from build123d import *

# Parameters (mm, degrees)
SKETCH_2_R      = 2
EXTRUDE_1_DEPTH = 5


with BuildPart() as part:
    # 草图2 → 凸台-拉伸1 (new, symmetric)
    with BuildSketch(Plane.XY):
        with BuildLine():
            ThreePointArc((18.5, 0), (15.999089719, 4.330652442), (10.99817977, 4.329075598))
            Line((10.99817977, 4.329075598), (2.50182023, 19.030924402))
            ThreePointArc((2.50182023, 19.030924402), (-1.295110422, 28.189356996), (0, 18.36))
            Line((0, 18.36), (0, 0))
            Line((0, 0), (-51.636977369, 0))
            Line((-51.636977369, 0), (-51.636977369, -8.430841873))
            Line((-51.636977369, -8.430841873), (41.612216194, -8.430841873))
            Line((41.612216194, -8.430841873), (41.612216194, 0))
            Line((41.612216194, 0), (18.5, 0))
        make_face()
        with BuildLine():
            ThreePointArc((15.280750547, 0), (13.5, -1.780750547), (11.719249453, 0))
            ThreePointArc((11.719249453, 0), (13.5, 1.780750547), (15.280750547, 0))
        make_face(mode=Mode.SUBTRACT)
        with Locations((0, 23.36)):
            Circle(SKETCH_2_R, mode=Mode.SUBTRACT)
    extrude(amount=EXTRUDE_1_DEPTH, both=True)


solid = part.part
The listing builds one solid part. Answer for the finished solid, in the listing's coordinates (mm). A direction names the side the tool comes from. Round coordinates to 2 decimals unless told otherwise and drop trailing zeros. Order: outer loops, then holes, each group sorted by start corner. A loop starts at its lowest first (then second) coordinate and runs counter-clockwise, first axis right, second up. Notation, with made-up numbers: (30.25, 69.5) - (39.25, 69.5) arc R17 cw to (39.25, 93.5) - close; hole circle Ø7 at (78.25, -19.5). An arc over 180 degrees is marked (long way). Write item = value, one per line. Start each with the question number.
1) For faces 1 (the flat face through (-2, -2, 5)), 2 (the flat face through (30, 0, 0)), 3 (the flat face through (0, 9, 0)), determine the directions among +Z, -Z, +X, -X, +Y, -Y from which every point of the face is accessible in a straight line to the end or side of a thin tool.
2) Section A-A, the plane z = -0.25 is taken. Write down the section's boundary in (x, y).
3) Straight lines are drawn through the part: L1, parallel to Y at x = 13.5, z = 0.25; L2, parallel to Y at x = -15.5, z = 1.5; L3, parallel to Y at x = -3.5, z = -0.75. For each, find the intervals that lie inside material, in ascending order.
4) Section B-B, the plane x = 13.5 is taken. Write down the section's boundary in (y, z).
5) For a pull along Y with two mould halves and no side action, classify faces 4 (the cylindrical face through (-1.099, 28.238, 0.07)), 5 (the flat face through (-2, -2, -5)), 6 (the flat face through (-6, -8.431, 0)) as released by +Y, released by -Y, zero draft, split by the parting line, or undercut.
6) Section D-D, the plane x = -20 is taken. Write down the section's boundary in (y, z).
7) Given pin 1 (1 mm diameter, centred on y = 6.5, z = -3, fed in from -X); pin 2 (5 mm diameter, centred on x = -25, z = -1, fed in from +Y); pin 3 (2 mm diameter, centred on x = 13.5, y = 0, fed in from -Z), each flat-ended and moving along its own axis, determine where each tip first touches the part or whether it passes through.
8) Section C-C, the plane y = 23.36 is taken. Write down the section's boundary in (x, z).
Results list:
q1.face_1 = +Z, +X, -X, +Y, -Y
q1.face_2 = +Z, -Z, +X, +Y
q1.face_3 = +Z, -Z, -X
q2.outline = (-51.64, -8.43) - (41.61, -8.43) - (41.61, 0) - (18.5, 0) arc R5 ccw to (11, 4.33) - (2.5, 19.03) arc R5 ccw (long way) to (0, 18.36) - (0, 0) - (-51.64, 0) - close; hole circle Ø4 at (0, 23.36); hole circle Ø3.56 at (13.5, 0)
q3.L1 = -8.43 to -1.78, 1.78 to 5
q3.L2 = -8.43 to 0
q3.L3 = -8.43 to 0, 19.79 to 26.93
q4.outline = (-8.43, -5) - (-1.78, -5) - (-1.78, 5) - (-8.43, 5) - close; (1.78, -5) - (5, -5) - (5, 5) - (1.78, 5) - close
q5.face_4 = undercut
q5.face_5 = zero draft
q5.face_6 = released by -Y
q6.outline = (-8.43, -5) - (0, -5) - (0, 5) - (-8.43, 5) - close
q7.pin_1 = 0
q7.pin_2 = 0
q7.pin_3 = through
q8.outline = (-5, -5) - (-2, -5) - (-2, 5) - (-5, 5) - close; (2, -5) - (5, -5) - (5, 5) - (2, 5) - close
